```python
from build123d import *

# Parameters (mm, degrees)
ESQUISSE1_R      = 2
ESQUISSE1_R_2    = 3
ESQUISSE1_R_3    = 10
ESQUISSE1_R_4    = 10.5
ESQUISSE1_R_5    = 2.000000001
ESQUISSE1_R_6    = 4
ESQUISSE1_R_7    = 1
ESQUISSE1_W      = 26
ESQUISSE1_H      = 60
ESQUISSE1_W_2    = 58
ESQUISSE1_H_2    = 4
ESQUISSE1_W_3    = 4
ESQUISSE1_H_3    = 9.5
EXTRUSION1_DEPTH = 3
CHANFREIN2_SIZE  = 3


with BuildPart() as part:
    # Esquisse1 → Extrusion1 (new body)
    with BuildSketch(Plane.XY):
        Polygon((-246.047840708, 39), (-186.047840708, -21), (-31.047840709, -21), (3.952159291, 14), (3.952159291, 169), (-56.047840709, 229), (-186.047840709, 229), (-246.047840708, 169), align=None)
        with Locations((-42.950847728, 11.872642083)):
            Circle(ESQUISSE1_R, mode=Mode.SUBTRACT)
        with Locations(Location((-1.12231419, 19.771416552, 0), (0, 0, 180))):
            Circle(ESQUISSE1_R_2, mode=Mode.SUBTRACT)
        with Locations((-36.022827062, -16)):
            Circle(ESQUISSE1_R_2, mode=Mode.SUBTRACT)
        with Locations((-28.808712104, 26.014777707)):
            Circle(ESQUISSE1_R, mode=Mode.SUBTRACT)
        with Locations((-203.319918647, 21.727922061)):
            Circle(ESQUISSE1_R_3, mode=Mode.SUBTRACT)
        with Locations(Location((-203.319918647, 7.585786438, 0), (0, 0, 180))):
            Circle(ESQUISSE1_R, mode=Mode.SUBTRACT)
        with Locations((-189.177783023, 21.727922061)):
            Circle(ESQUISSE1_R, mode=Mode.SUBTRACT)
        with Locations(Location((-203.319918647, 35.870057685, 0), (0, 0, 180))):
            Circle(ESQUISSE1_R, mode=Mode.SUBTRACT)
        with Locations((-28.808781353, 11.872704562)):
            Circle(ESQUISSE1_R_4, mode=Mode.SUBTRACT)
        with Locations((-217.462054271, 21.727922061)):
            Circle(ESQUISSE1_R, mode=Mode.SUBTRACT)
        with Locations(Location((-38.77576277, 172.129942315, 0), (0, 0, 180))):
            Circle(ESQUISSE1_R, mode=Mode.SUBTRACT)
        with Locations((-52.917898394, 186.272077939)):
            Circle(ESQUISSE1_R_5, mode=Mode.SUBTRACT)
        with Locations(Location((-38.77576277, 200.414213562, 0), (0, 0, 180))):
            Circle(ESQUISSE1_R, mode=Mode.SUBTRACT)
        with Locations((-24.633627146, 186.272077939)):
            Circle(ESQUISSE1_R, mode=Mode.SUBTRACT)
        with Locations((-38.77576277, 186.272077939)):
            Circle(ESQUISSE1_R_3, mode=Mode.SUBTRACT)
        with Locations(Location((-203.319918647, 186.272077939, 0), (0, 0, 180))):
            Circle(ESQUISSE1_R_3, mode=Mode.SUBTRACT)
        with Locations(Location((-217.462054271, 186.272077939, 0), (0, 0, 180))):
            Circle(ESQUISSE1_R, mode=Mode.SUBTRACT)
        with Locations((-203.319918647, 200.414213562)):
            Circle(ESQUISSE1_R, mode=Mode.SUBTRACT)
        with Locations(Location((-189.177783023, 186.272077939, 0), (0, 0, 180))):
            Circle(ESQUISSE1_R, mode=Mode.SUBTRACT)
        with Locations((-203.319918647, 172.129942315)):
            Circle(ESQUISSE1_R, mode=Mode.SUBTRACT)
        with Locations(Location((-182.221006385, -11.761204675, 0), (0, 0, 180))):
            Circle(ESQUISSE1_R_6, mode=Mode.SUBTRACT)
        with Locations((-182.221006385, 219.761204675)):
            Circle(ESQUISSE1_R_6, mode=Mode.SUBTRACT)
        with Locations((-236.809045383, 42.826834324)):
            Circle(ESQUISSE1_R_6, mode=Mode.SUBTRACT)
        with Locations((-5.047840709, 119.5)):
            Circle(ESQUISSE1_R, mode=Mode.SUBTRACT)
        with Locations(Location((-236.809045383, 165.173165676, 0), (0, 0, 180))):
            Circle(ESQUISSE1_R_6, mode=Mode.SUBTRACT)
        with Locations((-28.808712104, -2.269493541)):
            Circle(ESQUISSE1_R, mode=Mode.SUBTRACT)
        with Locations((-14.66657648, 11.872642083)):
            Circle(ESQUISSE1_R, mode=Mode.SUBTRACT)
        with Locations((-5.286636034, 165.173165676)):
            Circle(ESQUISSE1_R_6, mode=Mode.SUBTRACT)
        with Locations(Location((-59.874675032, 219.761204675, 0), (0, 0, 180))):
            Circle(ESQUISSE1_R_6, mode=Mode.SUBTRACT)
        with Locations(Location((-5.047840709, 88.5, 0), (0, 0, 180))):
            Circle(ESQUISSE1_R, mode=Mode.SUBTRACT)
        with Locations((-86.047840709, 136.5)):
            Circle(ESQUISSE1_R, mode=Mode.SUBTRACT)
        with Locations((-86.047840709, 122.5)):
            Circle(ESQUISSE1_R, mode=Mode.SUBTRACT)
        with Locations((-54.047840709, 119.5)):
            Circle(ESQUISSE1_R, mode=Mode.SUBTRACT)
        with Locations(Location((-54.047840709, 88.5, 0), (0, 0, 180))):
            Circle(ESQUISSE1_R, mode=Mode.SUBTRACT)
        with Locations((-46.022827062, 22)):
            Circle(ESQUISSE1_R_2, mode=Mode.SUBTRACT)
        with Locations((-121.047840709, 104)):
            Circle(ESQUISSE1_R_7, mode=Mode.SUBTRACT)
        Polygon((-192.047840709, 74), (-192.047840709, 84), (-184.047840709, 84), (-184.047840709, 93.5), (-192.047840709, 93.5), (-192.047840709, 134), (-218.047840709, 134), (-218.047840709, 104), (-218.047840709, 74), align=None, mode=Mode.SUBTRACT)
        with Locations((-37.047840709, 104)):
            Rectangle(ESQUISSE1_W, ESQUISSE1_H, mode=Mode.SUBTRACT)
        with Locations((-208.095681417, 143.5)):
            Rectangle(ESQUISSE1_W_2, ESQUISSE1_H_2, mode=Mode.SUBTRACT)
        with Locations((-235.095681417, 88.75)):
            Rectangle(ESQUISSE1_W_3, ESQUISSE1_H_3, mode=Mode.SUBTRACT)
    extrude(amount=EXTRUSION1_DEPTH)

    # Chanfrein2
    # the kernel refuses this chamfer: 3 mm, written as the material it takes off along each edge
    with BuildSketch(Plane(origin=(-46.022827062, 22, 0), x_dir=(1, 0, 0), z_dir=(0, -1, 0))) as chanfrein2_piece_1:
        Polygon((3, CHANFREIN2_SIZE), (3 + CHANFREIN2_SIZE, 0), (3, 0), align=None)
    revolve(axis=Axis((-46.022827062, 22, 0), (0, 0, 1)), mode=Mode.SUBTRACT)
    with BuildSketch(Plane(origin=(-36.022827062, -16, 0), x_dir=(1, 0, 0), z_dir=(0, -1, 0))) as chanfrein2_piece_2:
        Polygon((3, CHANFREIN2_SIZE), (3 + CHANFREIN2_SIZE, 0), (3, 0), align=None)
    revolve(axis=Axis((-36.022827062, -16, 0), (0, 0, 1)), mode=Mode.SUBTRACT)
    with BuildSketch(Plane(origin=(-1.12231419, 19.771416552, 0), x_dir=(-1, 0, 0), z_dir=(0, 1, 0))) as chanfrein2_piece_3:
        Polygon((3, CHANFREIN2_SIZE), (3 + CHANFREIN2_SIZE, 0), (3, 0), align=None)
    revolve(axis=Axis((-1.12231419, 19.771416552, 0), (0, 0, 1)), mode=Mode.SUBTRACT)


solid = part.part
```
Check sheet for the modelled part. Datum: model origin and axes. Units: mm. Coordinates: 2 decimals unless noted, no trailing zeros. Write each loop counter-clockwise with the first axis right and the second up, starting at its lowest first coordinate (ties: lowest second). Pieces come first, ordered by that corner, then holes. Notation, with made-up numbers: M 42.25,-6.5 L 101.25,-6.5 A32 cw 101.25,22.5 Z; hole C 25,27.25 d3. An arc over 180 degrees is marked long. Use one line per item in the form item = value.
Item 1: Material ranges on L1, parallel to X at y = 100.5, z = 2.95; L2, parallel to X at y = 88.5, z = 1.4; L3, parallel to Y at x = -183, z = 1.95, recorded low to high. Write a range as from..to.
Answer below:
L1 = -246.05..-218.05, -192.05..-50.05, -24.05..3.95
L2 = -246.05..-237.1, -233.1..-218.05, -184.05..-56.05, -52.05..-50.05, -24.05..-7.05, -3.05..3.95
L3 = -21..-15.68, -7.84..141.5, 145.5..215.84, 223.68..229
Item 2: Sectioned sample at A-A, the plane y = 114. Record the cut outline in (x, z), and give its area (3 significant figures).
Answer below:
outline = M -246.05,0 L -218.05,0 L -218.05,3 L -246.05,3 Z; M -192.05,0 L -50.05,0 L -50.05,3 L -192.05,3 Z; M -24.05,0 L 3.95,0 L 3.95,3 L -24.05,3 Z
area = 594 mm^2
Item 3: Release check for a two-part mould opening along Y. For faces 1 (the face through (-123, 106, 0)), 2 (the face through (-18.794, 15.027, 1.479)), 3 (the face through (-216.47, 9.42, 1.48)) record: pulls with the +Y half, pulls with the -Y half, needs draft (parallel to the pull), parting line crosses it, or undercut.
Answer below:
face_1 = needs draft
face_2 = undercut
face_3 = pulls with the -Y half
Item 4: Gauge pin test, flat ends, axial feed: pin 1 Ø6.5 at (x, y) = (-86.05, 122.5) entering from -Z; pin 2 Ø2.5 at (x, y) = (-52.92, 186.27) entering from -Z; pin 3 Ø1.5 at (y, z) = (193.5, 2) entering from +X. Record the tip position at first contact, or that the pin passes through.
Answer below:
pin_1 = 0
pin_2 = through
pin_3 = -19.8
Item 5: Sectioned sample at B-B, the plane z = 2.3. State how many separate pieces and enclosed holes the cut face has, and give its area (3 significant figures).
Answer below:
separate_pieces = 1
enclosed_holes = 40
area = 51,000 mm^2
